Here's the drawing with two shaded views (mm, measured from the low corner). I have some questions. A direction names the side the tool comes from. Round coordinates to 2 decimals unless told otherwise and drop trailing zeros. Order: outer loops, then holes, each group sorted by start corner. A loop starts at its lowest first (then second) coordinate and runs counter-clockwise, first axis right, second up. Notation, with made-up numbers: (68.25, 79.25) -> (105.25, 79.25) arc R21 cw to (105.25, 96.25) -> close; hole circle Ø10 at (-29.5, 47). An arc over 180 degrees is marked (long way). Use a Markdown table: item, result. Add a question column.
Q1. If we section it at A-A on y = 31: List the corners of the cut face in (x, z) for me (1 decimal).
Q2. For the marked faces 4, 5 and 6, which set-ups out of +Z, -Z, +X, -X, +Y, -Y let a thin tool reach every point of the face, with its end or its side?
Q3. If we section it at B-B on z = 3.25: List the corners of the cut face in (x, y) for me (1 decimal), plus the area to 3 significant figures.
Q4. I need wall thicknesses on line 1 along X through (y, z) = (43, 3.25) (1 decimal); line 2 along Y through (x, z) = (22, 9.75) (1 decimal); line 3 along Z through (x, y) = (7.5, 30.5). Which ranges of each line are inside material? Lowest first, please. Write a range as [from, to].
Q5. We'd pull the mould along Y, two halves only. Please class the marked faces 1, 2 and 3: +Y half, -Y half, draft (parallel to the pull), parting line (faces both ways), or undercut.
Q6. I'm going to push a flat-ended pin straight in: pin 1 Ø2 at (x, y) = (9, 71) entering from +Z. Where does the tip first touch, or does it pass through?
Q7. If we section it at D-D on z = 22.25: List the corners of the cut face in (x, y) for me (1 decimal).
Q8. If we section it at C-C on x = 13.5: List the corners of the cut face in (y, z) for me.
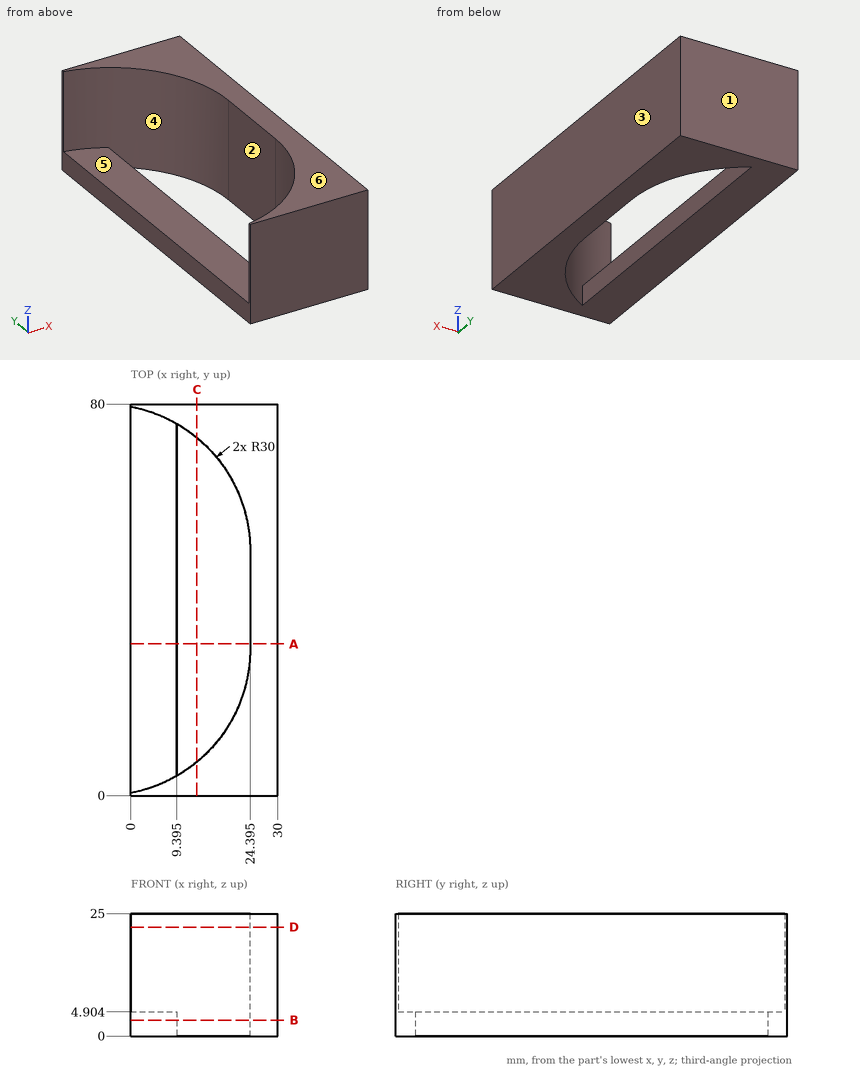
Answer below:
| question | item | result |
|---|---|---|
| 1 | outline | (0, 0) -> (9.4, 0) -> (9.4, 4.9) -> (0, 4.9) -> close; (24.4, 0) -> (30, 0) -> (30, 25) -> (24.4, 25) -> close |
| 2 | face 4 | +Z |
| 2 | face 5 | +Z, -X |
| 2 | face 6 | +Z, +X, -X, +Y, -Y |
| 3 | outline | (0, 0) -> (30, 0) -> (30, 80) -> (0, 80) -> close; hole (9.4, 4) arc R30 ccw to (24.4, 30) -> (24.4, 50) arc R30 ccw to (9.4, 76) -> close |
| 3 | area | 1,550 mm² |
| 4 | line 1 | [0, 9.4], [24.4, 30] |
| 4 | line 2 | [0, 18.3], [61.7, 80] |
| 4 | line 3 | [0, 4.9] |
| 5 | face 1 | +Y half |
| 5 | face 2 | undercut |
| 5 | face 3 | draft |
| 6 | pin 1 | z = 4.9 |
| 7 | outline | (0, 0) -> (30, 0) -> (30, 80) -> (0, 80) -> (0, 79.5) arc R30 cw to (24.4, 50) -> (24.4, 30) arc R30 cw to (0, 0.5) -> close |
| 8 | outline | (0, 0) -> (6.87, 0) -> (6.87, 25) -> (0, 25) -> close; (73.13, 0) -> (80, 0) -> (80, 25) -> (73.13, 25) -> close |
